Answer from the drawing. Dimensions are ordinates in mm from the lowest x, y and z of the part. A direction names the side the tool comes from. Give positions to 0.01 mm unless a question says otherwise; leave off trailing zeros. Write each loop counter-clockwise with the first axis right and the second up, starting at its lowest first coordinate (ties: lowest second). Pieces come first, ordered by that corner, then holes. Notation, with made-up numbers: M 66.5,63.25 L 125.5,63.25 A24 cw 125.5,93.25 Z; hole C 54,-16.5 d6. An arc over 180 degrees is marked long. Put each result on its own line as item: value.
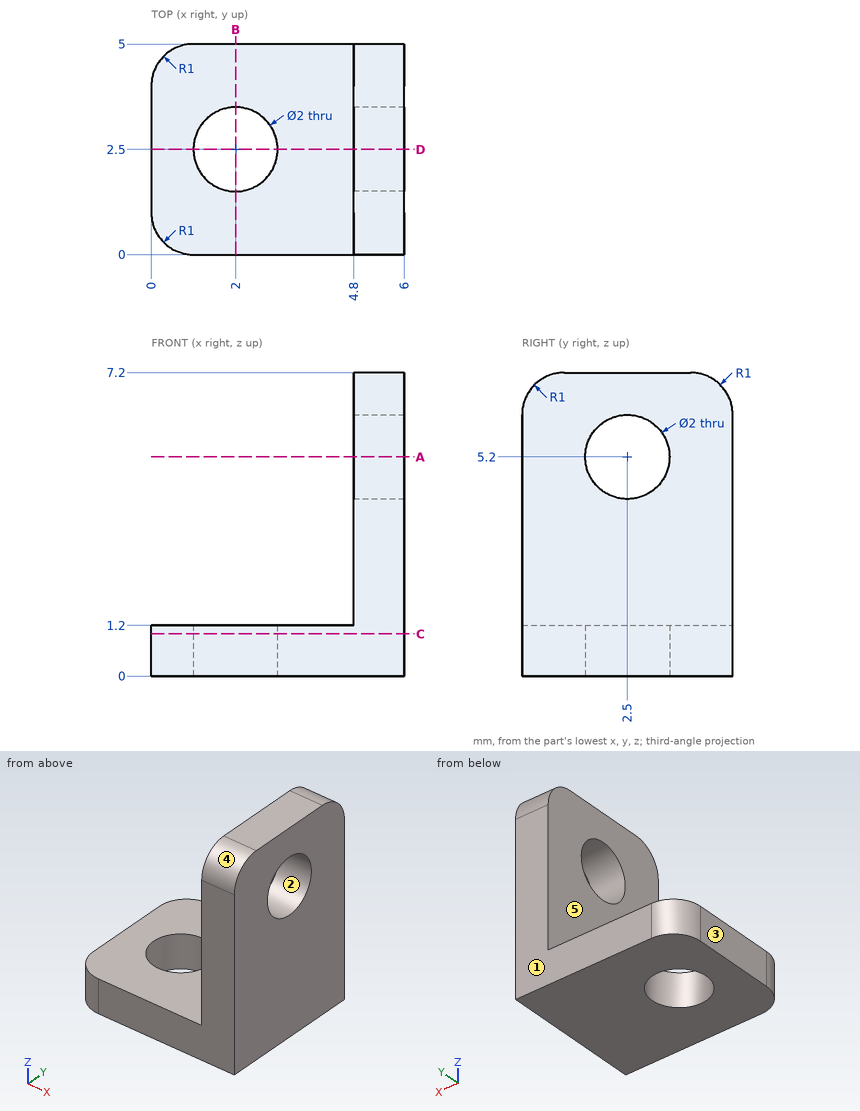
(1) Given pin 1 Ø3 at (x, y) = (2, 2.5) entering from +Z; pin 2 Ø2 at (x, z) = (3.5, 1.5) entering from +Y; pin 3 Ø1.5 at (y, z) = (3.5, 3) entering from -X, each flat-ended and moving along its own axis, determine where each tip first touches the part or whether it passes through.
Result:
pin 1: stops at z = 1.2
pin 2: stops at y = 5
pin 3: stops at x = 4.8
(2) Which of the six approach directions +Z, -Z, +X, -X, +Y, -Y give full straight-line access (tool end or side, diameter ignored) to the marked faces 4 and 5?
Result:
face 4: +Z, +X, -X, -Y
face 5: +Z, -X, +Y, -Y
(3) Straight lines are drawn through the part: line 1 along Y through (x, z) = (2, 0.45); line 2 along X through (y, z) = (4.45, 5.5); line 3 along Y through (x, z) = (5.5, 4.75). For each, find the intervals that lie inside material, in ascending order. Write a range as from..to.
Result:
line 1: y = 0..1.5, 3.5..5
line 2: x = 4.8..6
line 3: y = 0..1.61, 3.39..5
(4) Section C-C on z = 1 is taken. Determine the outline of the cut face in (x, y), and give its area (3 significant figures).
Result:
outline: M 0,1 A1 ccw 1,0 L 6,0 L 6,5 L 1,5 A1 ccw 0,4 Z; hole C 2,2.5 d2
area: 26.4 mm²
(5) Section A-A on z = 5.2 is taken. Determine the outline of the cut face in (x, y).
Result:
outline: M 4.8,0 L 6,0 L 6,1.5 L 4.8,1.5 Z; M 4.8,3.5 L 6,3.5 L 6,5 L 4.8,5 Z
(6) For a pull along Y with two mould halves and no side action, classify the marked faces 1, 2 and 3 as +Y half, -Y half, draft (parallel to the pull), parting line (faces both ways), or undercut.
Result:
face 1: +Y half
face 2: undercut
face 3: draft
(7) Section D-D on y = 2.5 is taken. Determine the outline of the cut face in (x, z), and give its area (3 significant figures).
Result:
outline: M 0,0 L 1,0 L 1,1.2 L 0,1.2 Z; M 3,0 L 6,0 L 6,4.2 L 4.8,4.2 L 4.8,1.2 L 3,1.2 Z; M 4.8,6.2 L 6,6.2 L 6,7.2 L 4.8,7.2 Z
area: 9.60 mm²
(8) Section B-B on x = 2 is taken. Determine the outline of the cut face in (y, z).
Result:
outline: M 0,0 L 1.5,0 L 1.5,1.2 L 0,1.2 Z; M 3.5,0 L 5,0 L 5,1.2 L 3.5,1.2 Z
